```python
from build123d import *

# Parameters (mm, degrees)
SKETCH1_R           = 35
BOSS_EXTRUDE1_DEPTH = 6
SKETCH11_W          = 10
SKETCH11_H          = 10
CUT_EXTRUDE3_DEPTH  = 3
SKETCH12_R          = 3.4
CUT_EXTRUDE4_DEPTH  = 50.859803449
SKETCH6_W           = 6.2
SKETCH6_H           = 6.2
CUT_EXTRUDE6_DEPTH  = 1.5


with BuildPart() as part:
    # Sketch1 → Boss-Extrude1 (new body)
    with BuildSketch(Plane(origin=(0, 0, 0), x_dir=(1, 0, 0), z_dir=(0, 1, 0))):
        with Locations(Location((0, 0, 0), (0, 0, 270))):
            Circle(SKETCH1_R)
    extrude(amount=BOSS_EXTRUDE1_DEPTH)

    # Sketch11 → Cut-Extrude3 (cut)
    with BuildSketch(Plane(origin=(0, 6, 0), x_dir=(1, 0, 0), z_dir=(0, 1, 0))):
        Rectangle(SKETCH11_W, SKETCH11_H)
    extrude(amount=-CUT_EXTRUDE3_DEPTH, mode=Mode.SUBTRACT)

    # Sketch12 → Cut-Extrude4 (cut, through all)
    with BuildSketch(Plane.XZ):
        with Locations(Location((15, -15, 0), (0, 0, 270))):
            Circle(SKETCH12_R)
        with Locations(Location((-15, -15, 0), (0, 0, 270))):
            Circle(SKETCH12_R)
        with Locations(Location((15, 15, 0), (0, 0, 270))):
            Circle(SKETCH12_R)
        with Locations(Location((-15, 15, 0), (0, 0, 270))):
            Circle(SKETCH12_R)
    extrude(amount=-CUT_EXTRUDE4_DEPTH, mode=Mode.SUBTRACT)

    # Sketch6 → Cut-Extrude6 (cut)
    with BuildSketch(Plane(origin=(0, 0, -4.132474232), x_dir=(1, 0, 0), z_dir=(0, -1, 0))):
        with Locations((-23.099150513, 4.136022025)):
            Rectangle(SKETCH6_W, SKETCH6_H)
        with Locations((0.003547793, 27.231624745)):
            Rectangle(SKETCH6_W, SKETCH6_H)
        with Locations((-0.003547793, -18.966676281)):
            Rectangle(SKETCH6_W, SKETCH6_H)
        with Locations((23.099150513, 4.128926439)):
            Rectangle(SKETCH6_W, SKETCH6_H)
    extrude(amount=-CUT_EXTRUDE6_DEPTH, mode=Mode.SUBTRACT)


solid = part.part
```
For this review, take the finished solid that the model builds, in its own axes (mm). A direction names the side the tool comes from. Coordinates: 2 decimals unless noted, no trailing zeros. Write each loop counter-clockwise with the first axis right and the second up, starting at its lowest first coordinate (ties: lowest second). Pieces come first, ordered by that corner, then holes.
(1) The part is to be moulded in two halves that separate along Z. For faces 4 (the face through (-21, 3, -28)), 5 (the face through (0, 0, 0)), 6 (the face through (-19.999, 1, 0)), say which applies: +Z half, -Z half, draft (parallel to the pull), parting line (faces both ways), or undercut.
(2) Add section D-D on x = 0. Give the boundary of the cut face in (y, z), then the cut area to 3 significant figures.
(3) For pin 1 Ø2 at (x, y) = (-8, 3.5) entering from +Z; pin 2 Ø1.9 at (x, z) = (21.5, 1) entering from -Y; pin 3 Ø0.8 at (x, y) = (22, 0.5) entering from -Z, all flat-tipped, find the tip position at first contact; note any pin that passes through.
(4) Wall thickness on probe 1 along X at (y, z) = (3.05, 15); probe 2 along Z at (x, y) = (-0.5, 1.6); probe 3 along Z at (x, y) = (-17, 2.5): over which ranges is each line inside the solid? List them lowest first.
(5) Tool access review of faces 1 (the face through (11.68, 2.96, 15.74)), 2 (the face through (0, 5, -5)), 3 (the face through (-23, 1, -3.096)): name each direction out of +Z, -Z, +X, -X, +Y, -Y from which nothing blocks a thin tool from reaching the whole face with its end or side.
(6) Add section B-B on x = 15. Give the boundary of the cut face in (y, z).
(7) Add section C-C on z = -16. Give the boundary of the cut face in (x, y), then the cut area to 3 significant figures.
(8) Add section A-A on y = 3.85. Give the boundary of the cut face in (x, z), then the cut area to 3 significant figures.
Answer sheet:
1. face 4: parting line
1. face 5: draft
1. face 6: undercut
2. outline: (0, -35) - (6, -35) - (6, -5) - (3, -5) - (3, 5) - (6, 5) - (6, 35) - (0, 35) - (0, 26.2) - (1.5, 26.2) - (1.5, 20) - (0, 20) - (0, -20) - (1.5, -20) - (1.5, -26.2) - (0, -26.2) - close
2. area: 371 mm2
3. pin 1: stops at z = 34.29
3. pin 2: stops at y = 1.5
3. pin 3: stops at z = -27.54
4. probe 1: x = -31.62 to -18.4, -11.6 to 11.6, 18.4 to 31.62
4. probe 2: z = -35 to 35
4. probe 3: z = -30.59 to -17.75, -12.25 to 12.25, 17.75 to 30.59
5. face 1: +Y, -Y
5. face 2: +Y
5. face 3: -Y
6. outline: (0, -31.62) - (6, -31.62) - (6, -18.4) - (0, -18.4) - close; (0, -11.6) - (6, -11.6) - (6, 11.6) - (0, 11.6) - close; (0, 18.4) - (6, 18.4) - (6, 31.62) - (0, 31.62) - close
7. outline: (-31.13, 0) - (-18.25, 0) - (-18.25, 6) - (-31.13, 6) - close; (-11.75, 0) - (11.75, 0) - (11.75, 6) - (-11.75, 6) - close; (18.25, 0) - (31.13, 0) - (31.13, 6) - (18.25, 6) - close
7. area: 296 mm2
8. outline: circle Ø70 at (0, 0); hole circle Ø6.8 at (-15, -15); hole circle Ø6.8 at (-15, 15); hole (-5, -5) - (5, -5) - (5, 5) - (-5, 5) - close; hole circle Ø6.8 at (15, -15); hole circle Ø6.8 at (15, 15)
8. area: 3,600 mm2
